Source: CAD feature listing. Evaluate the final solid. Frame: model axes, mm. A direction names the side the tool comes from. Round coordinates to 2 decimals unless told otherwise and drop trailing zeros. Loops run counter-clockwise (first coordinate to the right, second up) from the corner with the lowest first, then second, coordinate; pieces in that order, holes last. Notation, with made-up numbers: (10, 73.5) - (67, 73.5) arc R26 cw to (67, 105.5) - close; hole circle Ø5 at (88.5, -19). An arc over 180 degrees is marked (long way). One line per question, with ' | ' between items.
from build123d import *

# Parameters (mm, degrees)
SKETCH1_W           = 42
SKETCH1_H           = 42
BOSS_EXTRUDE1_DEPTH = 11
CHAMFER1_SIZE       = 3
CUT_EXTRUDE2_REACH  = 33.67
SKETCH3_R           = 1.5
SKETCH4_R           = 2.85
CUT_EXTRUDE3_DEPTH  = 3
SKETCH5_W           = 6
SKETCH5_H           = 7
CUT_EXTRUDE4_DEPTH  = 5


with BuildPart() as part:
    # Sketch1 → Boss-Extrude1 (new body)
    with BuildSketch(Plane.XY):
        Rectangle(SKETCH1_W, SKETCH1_H)
    extrude(amount=BOSS_EXTRUDE1_DEPTH)

    # Chamfer1
    chamfer1_edges = [part.edges().sort_by_distance(p)[0] for p in [
        (-21, 21, 5.5),
        (21, 21, 5.5),
        (21, -21, 5.5),
        (-21, -21, 5.5),
    ]]
    chamfer(chamfer1_edges, length=CHAMFER1_SIZE)

    # Sketch3 → Cut-Extrude2 (cut, up to next)
    with BuildSketch(Plane(origin=(0, 0, 0), x_dir=(-1, 0, 0), z_dir=(0, 0, -1)), mode=Mode.PRIVATE) as cut_extrude2_sk1:
        with Locations((-15.5, 15.5)):
            Circle(SKETCH3_R)
    cut_extrude2_tool1 = extrude(cut_extrude2_sk1.sketch, amount=-CUT_EXTRUDE2_REACH, mode=Mode.PRIVATE) & part.part
    # Sketch3 → Cut-Extrude2 (cut, up to next)
    with BuildSketch(Plane(origin=(0, 0, 0), x_dir=(-1, 0, 0), z_dir=(0, 0, -1)), mode=Mode.PRIVATE) as cut_extrude2_sk2:
        with Locations((15.5, 15.5)):
            Circle(SKETCH3_R)
    cut_extrude2_tool2 = extrude(cut_extrude2_sk2.sketch, amount=-CUT_EXTRUDE2_REACH, mode=Mode.PRIVATE) & part.part
    # Sketch3 → Cut-Extrude2 (cut, up to next)
    with BuildSketch(Plane(origin=(0, 0, 0), x_dir=(-1, 0, 0), z_dir=(0, 0, -1)), mode=Mode.PRIVATE) as cut_extrude2_sk3:
        with Locations((15.5, -15.5)):
            Circle(SKETCH3_R)
    cut_extrude2_tool3 = extrude(cut_extrude2_sk3.sketch, amount=-CUT_EXTRUDE2_REACH, mode=Mode.PRIVATE) & part.part
    # Sketch3 → Cut-Extrude2 (cut, up to next)
    with BuildSketch(Plane(origin=(0, 0, 0), x_dir=(-1, 0, 0), z_dir=(0, 0, -1)), mode=Mode.PRIVATE) as cut_extrude2_sk4:
        with Locations((-15.5, -15.5)):
            Circle(SKETCH3_R)
    cut_extrude2_tool4 = extrude(cut_extrude2_sk4.sketch, amount=-CUT_EXTRUDE2_REACH, mode=Mode.PRIVATE) & part.part
    add(cut_extrude2_tool1.solids().sort_by_distance((15.5, 15.5, 0))[0], mode=Mode.SUBTRACT)
    add(cut_extrude2_tool2.solids().sort_by_distance((-15.5, 15.5, 0))[0], mode=Mode.SUBTRACT)
    add(cut_extrude2_tool3.solids().sort_by_distance((-15.5, -15.5, 0))[0], mode=Mode.SUBTRACT)
    add(cut_extrude2_tool4.solids().sort_by_distance((15.5, -15.5, 0))[0], mode=Mode.SUBTRACT)

    # Sketch4 → Cut-Extrude3 (cut)
    with BuildSketch(Plane(origin=(0, 0, 0), x_dir=(-1, 0, 0), z_dir=(0, 0, -1))):
        with Locations((-15.5, 15.5)):
            Circle(SKETCH4_R)
        with Locations((15.5, 15.5)):
            Circle(SKETCH4_R)
        with Locations((15.5, -15.5)):
            Circle(SKETCH4_R)
        with Locations((-15.5, -15.5)):
            Circle(SKETCH4_R)
    extrude(amount=-CUT_EXTRUDE3_DEPTH, mode=Mode.SUBTRACT)

    # Sketch5 → Cut-Extrude4 (cut)
    with BuildSketch(Plane.XZ.offset(21)):
        with Locations((0, 7.5)):
            Rectangle(SKETCH5_W, SKETCH5_H)
    extrude(amount=-CUT_EXTRUDE4_DEPTH, mode=Mode.SUBTRACT)


solid = part.part
1. Section query D-D, the plane z = 6. Return loops of the section in (x, y), plus the area to 3 significant figures.
Worked out:
outline: (-21, -18) - (-18, -21) - (-3, -21) - (-3, -16) - (3, -16) - (3, -21) - (18, -21) - (21, -18) - (21, 18) - (18, 21) - (-18, 21) - (-21, 18) - close; hole circle Ø3 at (-15.5, -15.5); hole circle Ø3 at (-15.5, 15.5); hole circle Ø3 at (15.5, -15.5); hole circle Ø3 at (15.5, 15.5) | area: 1,690 mm2
2. Access query for faces 1 (the flat face through (-19, 20, 5)), 2 (the flat face through (-17, -17, 3)), 3 (the flat face through (0, -19, 4)). Directions: +Z, -Z, +X, -X, +Y, -Y. A direction counts if a zero-diameter tool reaches every point of the face in a straight line with its end or side. Return the directions, or none.
Worked out:
face 1: +Z, -Z, -X, +Y | face 2: -Z | face 3: +Z, -Y
3. Contact query for flat-ended pins moving along their axis: P1, Ø1.5, axis at x = 0, y = -18.5, coming from the +Z side; P2, Ø5, axis at x = 15.5, y = 15.5, coming from the -Z side; P3, Ø9, axis at x = -15.5, y = -15.5, coming from the +Z side; P4, Ø1.5, axis at y = -19, z = 7.5, coming from the +X side. Output: stop coordinate, or through.
Worked out:
P1: stops at z = 4 | P2: stops at z = 3 | P3: stops at z = 11 | P4: stops at x = 20.75
4. Section query B-B, the plane z = 3.5. Return loops of the section in (x, y).
Worked out:
outline: (-21, -18) - (-18, -21) - (18, -21) - (21, -18) - (21, 18) - (18, 21) - (-18, 21) - (-21, 18) - close; hole circle Ø3 at (-15.5, -15.5); hole circle Ø3 at (-15.5, 15.5); hole circle Ø3 at (15.5, -15.5); hole circle Ø3 at (15.5, 15.5)
5. Material intervals for probe 1 along Y at (x, z) = (15.5, 7); probe 2 along Y at (x, z) = (15.5, 1.1); probe 3 along X at (y, z) = (17, 1.25), sorted ascending.
Worked out:
probe 1: y = -21 to -17, -14 to 14, 17 to 21 | probe 2: y = -21 to -18.35, -12.65 to 12.65, 18.35 to 21 | probe 3: x = -21 to -17.92, -13.08 to 13.08, 17.92 to 21
6. Section query A-A, the plane y = 15.5. Return loops of the section in (x, z), plus the area to 3 significant figures.
Worked out:
outline: (-21, 0) - (-18.35, 0) - (-18.35, 3) - (-17, 3) - (-17, 11) - (-21, 11) - close; (-14, 3) - (-12.65, 3) - (-12.65, 0) - (12.65, 0) - (12.65, 3) - (14, 3) - (14, 11) - (-14, 11) - close; (17, 3) - (18.35, 3) - (18.35, 0) - (21, 0) - (21, 11) - (17, 11) - close | area: 380 mm2
7. Mould query, pull axis Y, two halves, no side actions, for faces 4 (the cylindrical face through (-14, 15.57, 6.94)), 5 (the flat face through (-19, -20, 5)), 6 (the cylindrical face through (17, -15.43, 6.94)), 7 (the flat face through (0, 0, 0)). Classes: released by +Y, released by -Y, zero draft, split by the parting line, or undercut.
Worked out:
face 4: undercut | face 5: released by -Y | face 6: undercut | face 7: zero draft
